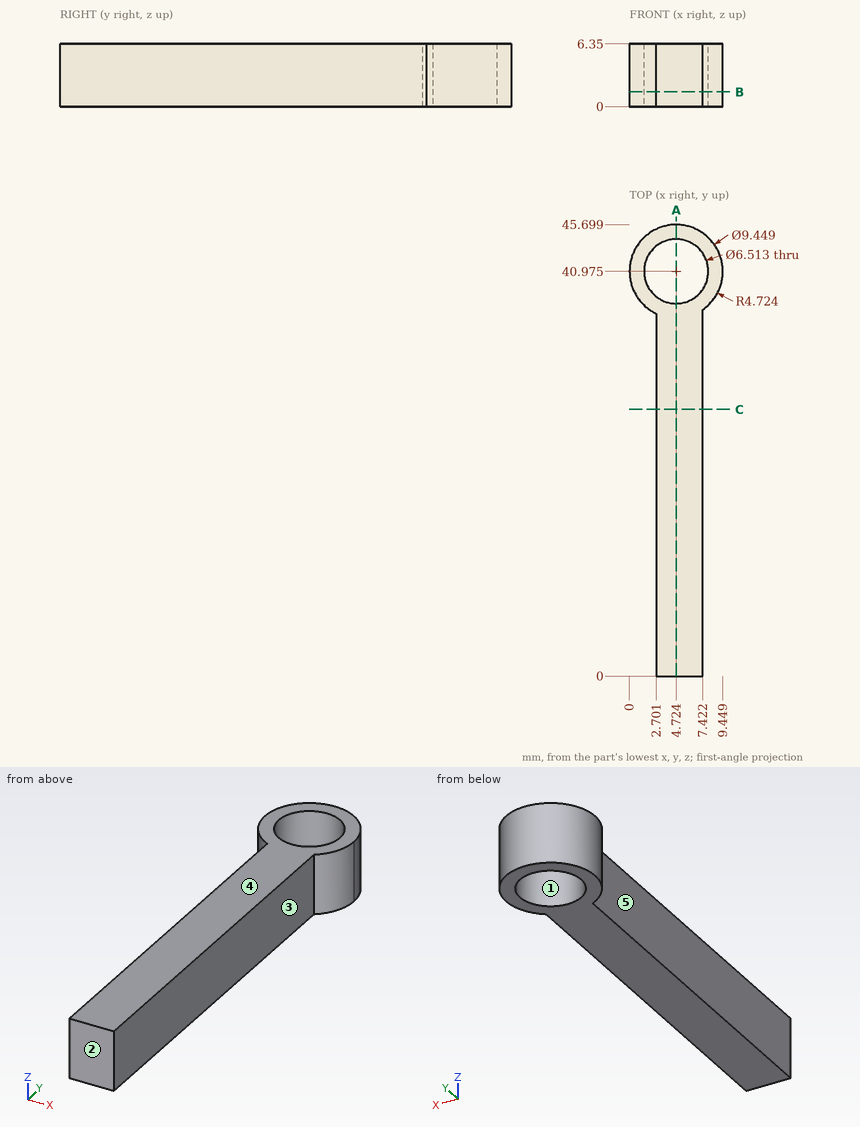
Geometry: see drawing. Coordinates: mm, zero at the bounding-box minimum. A direction names the side the tool comes from. Coordinates: 2 decimals unless noted, no trailing zeros. Loops run counter-clockwise (first coordinate to the right, second up) from the corner with the lowest first, then second, coordinate; pieces in that order, holes last. Notation, with made-up numbers: (-15.5, 47.25) - (14.5, 47.25) arc R3 cw to (14.5, 52.25) - close; hole circle Ø1 at (57.25, 32). An arc over 180 degrees is marked (long way). Put each result on its own line as item: value. Start each with the question number.
Q1. Cut plane A-A, the plane x = 4.75. Return loops of the section in (y, z).
Q2. Line query: line 1 (X direction, y = 32.5, z = 4.5); line 2 (Y direction, x = 2.5, z = 1) (1 decimal); line 3 (X direction, y = 43, z = 5) (1 decimal). Output: solid intervals per line, ascending.
Q3. Cut plane B-B, the plane z = 1.5. Return loops of the section in (x, y) (1 decimal).
Q4. Cut plane C-C, the plane y = 27. Return loops of the section in (x, z).
Q5. Pin query (flat end, axial travel): pin 1 Ø3 at (y, z) = (16, 3.5) entering from -X; pin 2 Ø3 at (y, z) = (8, 4) entering from +X; pin 3 Ø1.5 at (x, z) = (3.5, 4) entering from +Y (1 decimal). Return the tip coordinate at first contact, or that it passes through.
Q6. Pull-direction query (Y, two-part tool) for the marked faces 1, 2 and 3; classes: released by +Y, released by -Y, zero draft, split by the parting line, or undercut.
Q7. Set-up query: the marked faces 4 and 5. Return all of +Z, -Z, +X, -X, +Y, -Y with unobstructed straight access to the full face (end or side cutting, diameter ignored); none if empty.
Filled sheet:
1. outline: (0, 0) - (37.72, 0) - (37.72, 6.35) - (0, 6.35) - close; (44.23, 0) - (45.7, 0) - (45.7, 6.35) - (44.23, 6.35) - close
2. line 1: 2.7 to 7.42
2. line 2: 36.8 to 38.6, 43.4 to 45.1
2. line 3: 0.5 to 2.2, 7.3 to 9
3. outline: (2.7, 0) - (7.4, 0) - (7.4, 37.1) arc R4.7 ccw (long way) to (2.7, 36.7) - close; hole circle Ø6.5 at (4.7, 41)
4. outline: (2.7, 0) - (7.42, 0) - (7.42, 6.35) - (2.7, 6.35) - close
5. pin 1: x = 2.7
5. pin 2: x = 7.42
5. pin 3: y = 45.7
6. face 1: undercut
6. face 2: released by -Y
6. face 3: zero draft
7. face 4: +Z, +X, -X, +Y, -Y
7. face 5: +Z, -Z, -X, -Y
